Can you work these out from the model? Positions are in its coordinate system, mm. Round coordinates to 2 decimals unless told otherwise and drop trailing zeros. Loops run counter-clockwise (first coordinate to the right, second up) from the corner with the lowest first, then second, coordinate; pieces in that order, holes last.
(1) I want a section at B-B on x = 0. Write out the boundary of the cut face in (y, z) (3 decimals), plus the area to 3 significant figures.
(2) I want a section at A-A on z = 0. Write out the boundary of the cut face in (x, y) (3 decimals), plus the area to 3 significant figures.
(3) Will these pins go through, and if not, where does the flat tip stop? pin 1 Ø3 at (x, z) = (28.335, 0) entering from -Y; pin 2 Ø1.5 at (y, z) = (9, 18.5) entering from +X; pin 3 Ø3 at (y, z) = (8.5, 21.5) entering from +X; pin 4 Ø5 at (x, y) = (-7.5, 7) entering from -Z.
(4) I want a section at C-C on y = 6.5. Write out the boundary of the cut face in (x, z) (1 decimal), plus the area to 3 significant figures.
(5) If I drill on line 1 along X through (y, z) = (7.5, 0) (3 decimals); line 2 along X through (y, z) = (3, 10) (3 decimals); line 3 along Z through (x, y) = (30.5, 3), over which ranges is the centre line in solid material (lowest first)?
(6) Thinking about a two-plate mould opening in Z: for faces 1 (the face through (-36.525, 4.93, -8.111)), 2 (the face through (30.776, 4.93, -9.458)), 3 (the face through (1, 0, -1)), which applies, released by +Z, released by -Z, zero draft, split by the parting line, or undercut?
(7) I want a section at D-D on y = 2. Write out the boundary of the cut face in (x, z) (3 decimals), plus the area to 3 significant figures.
from build123d import *

# Parameters (mm, degrees)
SKETCH1_R           = 37.4142
SKETCH1_R_2         = 2.5
BOSS_EXTRUDE1_DEPTH = 10


with BuildPart() as part:
    # Sketch1 → Boss-Extrude1 (new body)
    with BuildSketch(Plane(origin=(0, 0, 0), x_dir=(1, 0, 0), z_dir=(0, 1, 0))):
        with Locations(Location((0, 0, 0), (0, 0, 270))):
            Circle(SKETCH1_R)
        with Locations(Location((-28.335, 0, 0), (0, 0, 270))):
            Circle(SKETCH1_R_2, mode=Mode.SUBTRACT)
        with Locations(Location((28.335, 0, 0), (0, 0, 90))):
            Circle(SKETCH1_R_2, mode=Mode.SUBTRACT)
        with Locations(Location((-28.335, 10, 0), (0, 0, 270))):
            Circle(SKETCH1_R_2, mode=Mode.SUBTRACT)
        with Locations(Location((-28.335, -10, 0), (0, 0, 270))):
            Circle(SKETCH1_R_2, mode=Mode.SUBTRACT)
        with Locations(Location((28.335, -10, 0), (0, 0, 90))):
            Circle(SKETCH1_R_2, mode=Mode.SUBTRACT)
        with Locations(Location((28.335, 10, 0), (0, 0, 90))):
            Circle(SKETCH1_R_2, mode=Mode.SUBTRACT)
    extrude(amount=BOSS_EXTRUDE1_DEPTH)

    # Sketch2 → Cut-Revolve12 (revolve, cut)
    with BuildSketch(Plane(origin=(0, 0, 0), x_dir=(0, 0, -1), z_dir=(1, 0, 0))):
        with BuildLine():
            Line((16.0792, 46.835), (16.0792, 4.165))
            ThreePointArc((16.0792, 4.165), (37.4142, 25.5), (16.0792, 46.835))
        make_face()
    revolve(axis=Axis((0, 52.533559147, -16.0792), (0, 1, 0)), mode=Mode.SUBTRACT)


solid = part.part
Filled sheet:
1. outline: (0, -37.414) - (10, -37.414) - (10, -30.74) arc R21.335 cw to (10, -1.419) - (10, 37.414) - (0, 37.414) - close
1. area: 631 mm2
2. outline: (-37.414, 0) - (-30.835, 0) - (-30.835, 10) - (-37.414, 10) - close; (-25.835, 0) - (25.835, 0) - (25.835, 10) - (-25.835, 10) - close; (30.835, 0) - (37.414, 0) - (37.414, 10) - (30.835, 10) - close
2. area: 648 mm2
3. pin 1: passes through
3. pin 2: stops at x = 32.94
3. pin 3: stops at x = 31.62
3. pin 4: stops at z = -37.08
4. outline: circle Ø74.8 at (0, 0); hole circle Ø5 at (-28.3, -10); hole circle Ø5 at (-28.3, 0); hole circle Ø5 at (-28.3, 10); hole circle Ø19.4 at (0, -16.1); hole circle Ø5 at (28.3, -10); hole circle Ø5 at (28.3, 0); hole circle Ø5 at (28.3, 10)
4. area: 3,980 mm2
5. line 1: x = -37.414 to -30.835, -25.835 to 25.835, 30.835 to 37.414
5. line 2: x = -36.053 to -30.835, -25.835 to 25.835, 30.835 to 36.053
5. line 3: z = -21.67 to -11.25, -8.75 to -1.25, 1.25 to 8.75, 11.25 to 21.67
6. face 1: split by the parting line
6. face 2: undercut
6. face 3: zero draft
7. outline: circle Ø74.828 at (0, 0); hole circle Ø5 at (-28.335, -10); hole circle Ø5 at (-28.335, 0); hole circle Ø5 at (-28.335, 10); hole circle Ø5 at (28.335, -10); hole circle Ø5 at (28.335, 0); hole circle Ø5 at (28.335, 10)
7. area: 4,280 mm2
